For this review, take the finished solid that the model builds, in its own axes (mm). Coordinates: 2 decimals unless noted, no trailing zeros. Write each loop counter-clockwise with the first axis right and the second up, starting at its lowest first coordinate (ties: lowest second). Pieces come first, ordered by that corner, then holes. Notation, with made-up numbers: M 70.25,8 L 96.25,8 A20 ccw 96.25,44 Z; hole C -39,-27.75 d9. An arc over 180 degrees is marked long. One line per question, with ' | ' between items.
from build123d import *

# Parameters (mm, degrees)
F0_W     = 72
F0_H     = 84
F0_R     = 1.5
F1_DEPTH = 2
F2_W     = 2
F2_H     = 8
F2_W_2   = 24
F3_DEPTH = 7
F4_W     = 24
F4_H     = 5
F5_DEPTH = 8
F6_R     = 1
F7_DEPTH = 5


with BuildPart() as f1:
    # F0 (on Top) → F1 (new body)
    with BuildSketch(Plane.XY):
        Rectangle(F0_W, F0_H)
        with Locations((-30.5, -36.5)):
            Circle(F0_R, mode=Mode.SUBTRACT)
        with Locations((30, -36.5)):
            Circle(F0_R, mode=Mode.SUBTRACT)
        with Locations((-30.5, 37)):
            Circle(F0_R, mode=Mode.SUBTRACT)
        with Locations((30, 37)):
            Circle(F0_R, mode=Mode.SUBTRACT)
    extrude(amount=F1_DEPTH)

    # F2 (on face) → F3 (join)
    with BuildSketch(Plane.XY.offset(2)):
        with Locations((-15, 20)):
            Rectangle(F2_W, F2_H)
        with Locations((-2, 20)):
            Rectangle(F2_W_2, F2_H)
        with Locations((11, 20)):
            Rectangle(F2_W, F2_H)
    extrude(amount=F3_DEPTH)

    # F4 (on face) → F5 (cut, through all)
    with BuildSketch(Plane.XZ.offset(-16)):
        with Locations((-2, 4.5)):
            Rectangle(F4_W, F4_H)
    extrude(amount=-F5_DEPTH, mode=Mode.SUBTRACT)

    # F6
    f6_edges = [f1.edges().sort_by_distance(p)[0] for p in [
        (-14, 20, 7),
        (10, 20, 7),
        (12, 20, 9),
        (-16, 20, 9),
        (-16, 20, 2),
        (-14, 20, 2),
        (10, 20, 2),
        (12, 20, 2),
    ]]
    fillet(f6_edges, radius=F6_R)

    # F2 (on face) → F7 (join)
    with BuildSketch(Plane.XY.offset(2)):
        Polygon((12, 8), (10, 8), (10, 0), (2, 0), (2, -2), (12, -2), align=None)
        Polygon((-14, 0), (-14, 8), (-16, 8), (-16, -2), (-6, -2), (-6, 0), align=None)
    extrude(amount=F7_DEPTH)


solid = f1.part
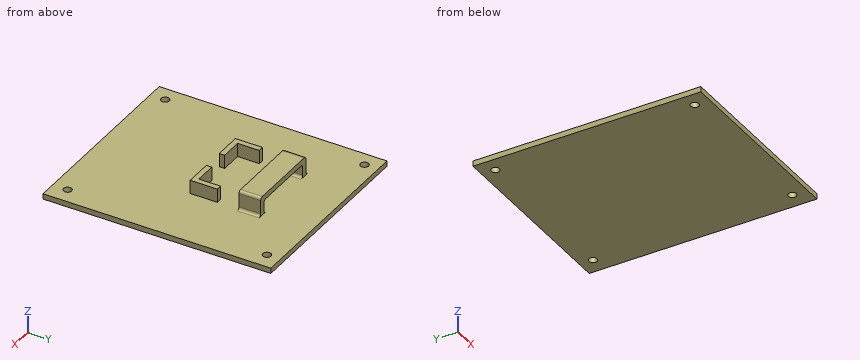
1) We need section A-A on x = -30.5. State the section outline as (y, z) points.
Responses:
outline: M -42,0 L -38,0 L -38,2 L -42,2 Z; M -35,0 L 35.5,0 L 35.5,2 L -35,2 Z; M 38.5,0 L 42,0 L 42,2 L 38.5,2 Z
2) We need section D-D on x = 17. State the section outline as (y, z) points, then the cut area to 3 significant figures.
Responses:
outline: M -42,0 L 42,0 L 42,2 L -42,2 Z | area: 168 mm^2
3) To check wall thickness, follow line 1 along Y through (x, z) = (30, 1.15); line 2 along Z through (x, y) = (-9.5, 20); line 3 along Z through (x, y) = (-18.5, -18). State the ranges of each line that lie inside material, in increasing order. Write a range as [from, to].
Responses:
line 1: [-42, -38], [-35, 35.5], [38.5, 42] | line 2: [0, 2], [7, 9] | line 3: [0, 2]
4) Insertion check: pin 1 Ø5 at (x, y) = (-30.5, -36.5) entering from +Z; pin 2 Ø2.5 at (x, z) = (8.5, 4) entering from -Y; pin 3 Ø2 at (x, z) = (-14.5, 5.5) entering from +Y. Each pin has a flat end and moves straight along its axis. Give the tip position at first contact, or say it passes through.
Responses:
pin 1: z = 2 | pin 2: y = -2 | pin 3: y = 24
5) We need section B-B on y = -36.5. State the section outline as (x, z) points, then the cut area to 3 significant figures.
Responses:
outline: M -36,0 L -32,0 L -32,2 L -36,2 Z; M -29,0 L 28.5,0 L 28.5,2 L -29,2 Z; M 31.5,0 L 36,0 L 36,2 L 31.5,2 Z | area: 132 mm^2
6) We need section C-C on x = 7.5. State the section outline as (y, z) points.
Responses:
outline: M -42,0 L 42,0 L 42,2 L 0,2 L 0,7 L -2,7 L -2,2 L -42,2 Z; M 16,7 L 24,7 L 24,9 L 16,9 Z
